Source: CAD feature listing. Evaluate the final solid. Frame: model axes, mm. Round coordinates to 2 decimals unless told otherwise and drop trailing zeros. Loops run counter-clockwise (first coordinate to the right, second up) from the corner with the lowest first, then second, coordinate; pieces in that order, holes last. Notation, with made-up numbers: (32.25, 63) - (81.25, 63) arc R16 ccw to (81.25, 84) - close; hole circle Ø5 at (80, -17.75). An arc over 180 degrees is marked (long way). One line per question, with ' | ' between items.
from build123d import *

# Parameters (mm, degrees)
F1_DEPTH = 1130.3
F2_R     = 2.35
F3_DEPTH = 25.4
F2_R_2   = 4
F4_DEPTH = 3.16
F5_SIZE  = 0.508


with BuildPart() as f1:
    # F0 (on Front) → F1 (new body)
    with BuildSketch(Plane.XZ):
        Polygon((-7.5311, -5.03968), (-7.5311, -7.278751), (7.5311, -7.278751), (7.5311, -5.03968), (6.868491, -5.03968), (6.868491, 0.495178), (7.5311, 0.495178), (7.5311, 3.355941), (6.916133, 3.970907), (5.987299, 3.970907), (5.987299, 5.026974), (6.916133, 5.026974), (7.5311, 5.641941), (7.5311, 7.351649), (-7.5311, 7.351649), (-7.5311, 5.641941), (-6.916133, 5.026974), (-5.987299, 5.026974), (-5.987299, 3.970907), (-6.916133, 3.970907), (-7.5311, 3.355941), (-7.5311, 0.495178), (-6.868491, 0.495178), (-6.868491, -5.03968), align=None)
    extrude(amount=F1_DEPTH)

    # F2 (on face) → F3 (cut)
    with BuildSketch(Plane.XY.offset(7.351649)):
        with Locations((0, -30.189795)):
            Circle(F2_R)
        with Locations((0, -90.189795)):
            Circle(F2_R)
        with Locations((0, -150.189795)):
            Circle(F2_R)
        with Locations((0, -210.189795)):
            Circle(F2_R)
        with Locations((0, -270.189795)):
            Circle(F2_R)
        with Locations((0, -330.189795)):
            Circle(F2_R)
        with Locations((0, -390.189795)):
            Circle(F2_R)
        with Locations((0, -450.189795)):
            Circle(F2_R)
        with Locations((0, -510.189795)):
            Circle(F2_R)
        with Locations((0, -570.189795)):
            Circle(F2_R)
        with Locations((0, -630.189795)):
            Circle(F2_R)
        with Locations((0, -690.189795)):
            Circle(F2_R)
        with Locations((0, -750.189795)):
            Circle(F2_R)
        with Locations((0, -810.189795)):
            Circle(F2_R)
        with Locations((0, -870.189795)):
            Circle(F2_R)
        with Locations((0, -930.189795)):
            Circle(F2_R)
        with Locations((0, -990.189795)):
            Circle(F2_R)
        with Locations((0, -1050.189795)):
            Circle(F2_R)
        with Locations((0, -1110.189795)):
            Circle(F2_R)
    extrude(amount=-F3_DEPTH, mode=Mode.SUBTRACT)

    # F2 (on face) → F4 (cut)
    with BuildSketch(Plane.XY.offset(7.351649)):
        with Locations((0, -1110.189795)):
            Circle(F2_R_2)
        with Locations((0, -1110.189795)):
            Circle(F2_R, mode=Mode.SUBTRACT)
        with Locations((0, -1050.189795)):
            Circle(F2_R_2)
        with Locations((0, -1050.189795)):
            Circle(F2_R, mode=Mode.SUBTRACT)
        with Locations((0, -990.189795)):
            Circle(F2_R_2)
        with Locations((0, -990.189795)):
            Circle(F2_R, mode=Mode.SUBTRACT)
        with Locations((0, -930.189795)):
            Circle(F2_R_2)
        with Locations((0, -930.189795)):
            Circle(F2_R, mode=Mode.SUBTRACT)
        with Locations((0, -870.189795)):
            Circle(F2_R_2)
        with Locations((0, -870.189795)):
            Circle(F2_R, mode=Mode.SUBTRACT)
        with Locations((0, -810.189795)):
            Circle(F2_R_2)
        with Locations((0, -810.189795)):
            Circle(F2_R, mode=Mode.SUBTRACT)
        with Locations((0, -750.189795)):
            Circle(F2_R_2)
        with Locations((0, -750.189795)):
            Circle(F2_R, mode=Mode.SUBTRACT)
        with Locations((0, -690.189795)):
            Circle(F2_R_2)
        with Locations((0, -690.189795)):
            Circle(F2_R, mode=Mode.SUBTRACT)
        with Locations((0, -630.189795)):
            Circle(F2_R_2)
        with Locations((0, -630.189795)):
            Circle(F2_R, mode=Mode.SUBTRACT)
        with Locations((0, -570.189795)):
            Circle(F2_R_2)
        with Locations((0, -570.189795)):
            Circle(F2_R, mode=Mode.SUBTRACT)
        with Locations((0, -510.189795)):
            Circle(F2_R_2)
        with Locations((0, -510.189795)):
            Circle(F2_R, mode=Mode.SUBTRACT)
        with Locations((0, -450.189795)):
            Circle(F2_R_2)
        with Locations((0, -450.189795)):
            Circle(F2_R, mode=Mode.SUBTRACT)
        with Locations((0, -390.189795)):
            Circle(F2_R_2)
        with Locations((0, -390.189795)):
            Circle(F2_R, mode=Mode.SUBTRACT)
        with Locations((0, -330.189795)):
            Circle(F2_R_2)
        with Locations((0, -330.189795)):
            Circle(F2_R, mode=Mode.SUBTRACT)
        with Locations((0, -270.189795)):
            Circle(F2_R_2)
        with Locations((0, -270.189795)):
            Circle(F2_R, mode=Mode.SUBTRACT)
        with Locations((0, -210.189795)):
            Circle(F2_R_2)
        with Locations((0, -210.189795)):
            Circle(F2_R, mode=Mode.SUBTRACT)
        with Locations((0, -150.189795)):
            Circle(F2_R_2)
        with Locations((0, -150.189795)):
            Circle(F2_R, mode=Mode.SUBTRACT)
        with Locations((0, -90.189795)):
            Circle(F2_R_2)
        with Locations((0, -90.189795)):
            Circle(F2_R, mode=Mode.SUBTRACT)
        with Locations((0, -30.189795)):
            Circle(F2_R_2)
        with Locations((0, -30.189795)):
            Circle(F2_R, mode=Mode.SUBTRACT)
    extrude(amount=-F4_DEPTH, mode=Mode.SUBTRACT)

    # F5
    f5_edges = [f1.edges().sort_by_distance(p)[0] for p in [
        (7.5311, -565.15, 7.351649),
        (0, 0, 7.351649),
        (0, -1130.3, 7.351649),
        (-7.5311, -565.15, 7.351649),
        (-4, -1110.189795, 7.351649),
        (-4, -1050.189795, 7.351649),
        (-4, -990.189795, 7.351649),
        (-4, -930.189795, 7.351649),
        (-4, -870.189795, 7.351649),
        (-4, -810.189795, 7.351649),
        (-4, -750.189795, 7.351649),
        (-4, -690.189795, 7.351649),
        (-4, -630.189795, 7.351649),
        (-4, -570.189795, 7.351649),
        (-4, -510.189795, 7.351649),
        (-4, -450.189795, 7.351649),
        (-4, -390.189795, 7.351649),
        (-4, -330.189795, 7.351649),
        (-4, -270.189795, 7.351649),
        (-4, -210.189795, 7.351649),
        (-4, -150.189795, 7.351649),
        (-4, -90.189795, 7.351649),
        (-4, -30.189795, 7.351649),
        (-7.5311, -565.15, -7.278751),
        (0, 0, -7.278751),
        (0, -1130.3, -7.278751),
        (7.5311, -565.15, -7.278751),
        (-2.35, -1110.189795, -7.278751),
        (-2.35, -1050.189795, -7.278751),
        (-2.35, -990.189795, -7.278751),
        (-2.35, -930.189795, -7.278751),
        (-2.35, -870.189795, -7.278751),
        (-2.35, -810.189795, -7.278751),
        (-2.35, -750.189795, -7.278751),
        (-2.35, -690.189795, -7.278751),
        (-2.35, -630.189795, -7.278751),
        (-2.35, -570.189795, -7.278751),
        (-2.35, -510.189795, -7.278751),
        (-2.35, -450.189795, -7.278751),
        (-2.35, -390.189795, -7.278751),
        (-2.35, -330.189795, -7.278751),
        (-2.35, -270.189795, -7.278751),
        (-2.35, -210.189795, -7.278751),
        (-2.35, -150.189795, -7.278751),
        (-2.35, -90.189795, -7.278751),
        (-2.35, -30.189795, -7.278751),
    ]]
    chamfer(f5_edges, length=F5_SIZE)


solid = f1.part
1. Contact query for flat-ended pins moving along their axis: P1, Ø3, axis at x = 0, y = -510.19, coming from the +Z side; P2, Ø5.5, axis at x = 0, y = -570.19, coming from the +Z side; P3, Ø5, axis at x = 0, y = -1050.19, coming from the -Z side. Output: stop coordinate, or through.
Worked out:
P1: passes through | P2: stops at z = 4.19 | P3: stops at z = -6.92
2. Section query A-A, the plane y = -711. Return loops of the section in (x, z).
Worked out:
outline: (-7.53, -6.77) - (-7.02, -7.28) - (7.02, -7.28) - (7.53, -6.77) - (7.53, -5.04) - (6.87, -5.04) - (6.87, 0.5) - (7.53, 0.5) - (7.53, 3.36) - (6.92, 3.97) - (5.99, 3.97) - (5.99, 5.03) - (6.92, 5.03) - (7.53, 5.64) - (7.53, 6.84) - (7.02, 7.35) - (-7.02, 7.35) - (-7.53, 6.84) - (-7.53, 5.64) - (-6.92, 5.03) - (-5.99, 5.03) - (-5.99, 3.97) - (-6.92, 3.97) - (-7.53, 3.36) - (-7.53, 0.5) - (-6.87, 0.5) - (-6.87, -5.04) - (-7.53, -5.04) - close
3. Material intervals for probe 1 along X at (y, z) = (-449.5, -0.5); probe 2 along X at (y, z) = (-539.5, -1.75); probe 3 along X at (y, z) = (-631, 3.5), sorted ascending.
Worked out:
probe 1: x = -6.87 to -2.25, 2.25 to 6.87 | probe 2: x = -6.87 to 6.87 | probe 3: x = -7.39 to -2.21, 2.21 to 7.39
4. Section query B-B, the plane x = 0. Give the number of separate pieces and of enclosed holes in the cut face, plus the area to 3 significant figures.
Worked out:
separate pieces: 20 | enclosed holes: 0 | area: 15,000 mm2
